Autodesk Inventor part; units mm, degrees
ref_plane "YZ Plane" through (0, 0, 0) normal (1, 0, 0) x (0, 1, 0)
ref_plane "XZ Plane" through (0, 0, 0) normal (0, 1, 0) x (-1, 0, 0)
ref_plane "XY Plane" through (0, 0, 0) normal (0, 0, 1) x (1, 0, 0)
sketch "Sketch2" plane through (0, 0, 0) normal (0, 0, 1) x (1, 0, 0)
  line L0 (9.5, 0) -> (9.5, -25.4)
  line L1 (9.5, 0) -> (28.535, 0)
  line L2 (9.5, -25.4) -> (26.985, -25.4)
  line L3 (28.535, 0) -> (26.985, -25.4)
  line L4 (0, -30.48) -> (0, 5.08)
  point P0 (0, 0)
  dimension "d5" = 9.5
  dimension "d6" = 25.4
  dimension "d7" = 19.035
  dimension "d8" = 17.485
revolve "Revolution1" add sketch "Sketch2" angle 358 mid plane about axis through (0, -10, 0) along (0, 1, 0)
sketch "Sketch3" plane through (0, 0, 0) normal (0, 1, 0) x (-1, 0, 0)
  line L0 (0, 0) -> (-7.055, 10.0756) construction
  line L1 (0, 0) -> (-9.5, 0) construction
  arc A0 (9.4986, 0.1658) -> (9.4986, -0.1658) centre (0, 0) ccw
  line L2 (-9.5124, 8.3548) -> (-4.5975, 11.7963)
  line L3 (-9.5124, 8.3548) -> (-7.6276, 5.663)
  line L4 (-4.5975, 11.7963) -> (-2.7127, 9.1045)
  dimension "d10" = 55
  dimension "d11" = 12.3
  dimension "d12" = 6
extrude "Extrusion2" cut sketch "Sketch3" against normal through all
sketch "Sketch4" plane through (0, 0, 0) normal (0, 1, 0) x (-1, 0, 0)
  arc A0 (26.9809, 0.471) -> (26.9809, -0.471) centre (0, 0) ccw
  point P0 (0, 0)
  point P1 (-26.985, 0)
sketch "Sketch5" plane through (0, 0, 0) normal (0, 1, 0) x (-1, 0, 0)
  arc A0 (26.9809, 0.471) -> (26.9809, -0.471) centre (0, 0) ccw
  arc A1 (26.9809, 0.471) -> (26.9809, -0.471) centre (0, 0) ccw
  line L0 (0, 0) -> (26.985, 0) construction
  line L1 (0, 0) -> (3.6164, 41.3358) construction
  line L2 (0, 0) -> (3.8154, -43.6107) construction
  point P0 (0, 0)
  point P1 (-26.6885, 3.989)
  point P2 (-26.6885, -3.989)
  point P3 (2.3519, -26.8823)
  point P4 (2.3519, 26.8823)
  dimension "d18" = 85
  dimension "d21" = 85
hole "Hole1" at (26.985, 0, 0) direction (0, -1, 0) diameter 8 end through all
hole "Hole2" at (-2.3519, 0, -26.8823) at (-2.3519, 0, 26.8823) direction (0, -1, 0) diameter 8 depth 15 tip angle 118
equation "\"d21\" = d18"
properties part number "Втулка для шкива"
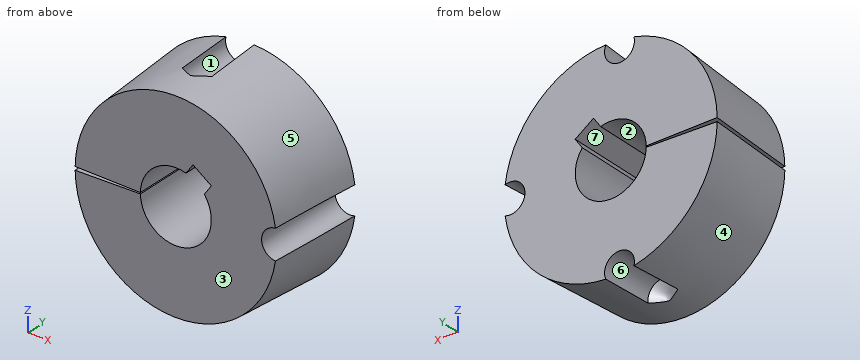
Geometry: final body of the model. Coordinates: model frame, mm. Face numbers are marked on the shaded views. A direction names the side the tool comes from. Round coordinates to 2 decimals unless told otherwise and drop trailing zeros. Order: outer loops, then holes, each group sorted by start corner. A loop starts at its lowest first (then second) coordinate and runs counter-clockwise, first axis right, second up.
Q1. Material intervals for probe 1 along X at (y, z) = (-21, -1.5); probe 2 along X at (y, z) = (-12.75, 0) (3 decimals); probe 3 along Z at (x, y) = (-5.5, -13.75), sorted ascending.
Result sheet:
probe 1: x = -27.21 to -9.38, 9.38 to 23.28
probe 2: x = 9.5 to 22.985
probe 3: z = -24.41 to -7.75, 7.75 to 24.41
Q2. Mould query, pull axis Z, two halves, no side actions, for the marked faces 4, 5, 6 and 7. Classes: released by +Z, released by -Z, zero draft, split by the parting line, or undercut.
Result sheet:
face 4: released by -Z
face 5: released by +Z
face 6: undercut
face 7: undercut
Q3. Section A-A, the plane y = -15.75. Output: boundary loops of the cut face in (x, z) (1 decimal).
Result sheet:
outline: (-27.6, -0.5) arc R27.6 ccw to (-5.1, -27.1) arc R2.8 cw (long way) to (0.3, -27.6) arc R27.6 ccw to (27.3, -4) arc R4 cw (long way) to (27.3, 4) arc R27.6 ccw to (0.3, 27.6) arc R2.8 cw (long way) to (-5.1, 27.1) arc R27.6 ccw to (-27.6, 0.5) - (-9.5, 0.2) arc R9.5 cw to (2.7, 9.1) - (4.6, 11.8) - (9.5, 8.4) - (7.6, 5.7) arc R9.5 cw (long way) to (-9.5, -0.2) - close
Q4. Access query for the marked faces 1, 2 and 3. Directions: +Z, -Z, +X, -X, +Y, -Y. A direction counts if a zero-diameter tool reaches every point of the face in a straight line with its end or side. Return the directions, or none.
Result sheet:
face 1: +Y
face 2: +Y, -Y
face 3: +Z, -Z, +X, -X, -Y
Q5. Pin query (flat end, axial travel): pin 1 (6 mm diameter, centred on x = -3, y = -11.5, fed in from +Z); pin 2 (4 mm diameter, centred on y = -10, z = 3.5, fed in from +X); pin 3 (6 mm diameter, centred on y = -10, z = -16.5, fed in from +X); pin 4 (5 mm diameter, centred on x = 26.985, z = 0, fed in from +Y). Return the tip coordinate at first contact, or that it passes through.
Result sheet:
pin 1: stops at z = 25.24
pin 2: stops at x = 27.77
pin 3: stops at x = 24.46
pin 4: passes through
